Could you check a few things on this model? Use its own coordinates, in mm. Coordinates: 2 decimals unless noted, no trailing zeros. Order: outer loops, then holes, each group sorted by start corner. A loop starts at its lowest first (then second) coordinate and runs counter-clockwise, first axis right, second up. Notation, with made-up numbers: (31.25, 62.25) -> (35.25, 62.25) arc R11 ccw to (35.25, 68.25) -> close; hole circle Ø6 at (-35.75, -1). An arc over 180 degrees is marked (long way). Use a Markdown table: item, result. Add a question column.
1) If we section it at C-C (z = -54.5): Write out the boundary of the cut face in (x, y), plus the area to 3 significant figures.
2) If we section it at B-B (x = 44): Write out the boundary of the cut face in (y, z).
3) If we section it at A-A (y = 0.8): Write out the boundary of the cut face in (x, z).
4) If I drill on L1, parallel to Z at x = 17, y = 1.85; L2, parallel to Z at x = 67.5, y = 2.3; L3, parallel to X at y = 0.5, z = 36.5, over which ranges is the centre line in solid material (lowest first)? Write a range as [from, to].
5) Will these pins go through, and if not, where does the flat tip stop? pin 1 Ø3.5 at (x, z) = (77, 0) entering from +Y; pin 2 Ø2.5 at (x, z) = (-39, 66.39) entering from -Y.
```python
from build123d import *

# Parameters (mm, degrees)
SKETCH1_R           = 75
SKETCH1_R_2         = 73.5
SKETCH1_R_3         = 1.5
BOSS_EXTRUDE1_DEPTH = 2.5


with BuildPart() as part:
    # Sketch1 → Boss-Extrude1 (new body)
    with BuildSketch(Plane(origin=(0, 0, 0), x_dir=(1, 0, 0), z_dir=(0, 1, 0))):
        Circle(SKETCH1_R)
        Circle(SKETCH1_R_2, mode=Mode.SUBTRACT)
        Circle(SKETCH1_R_2)
        with BuildLine():
            ThreePointArc((-65.092339325, -37.255702398), (-75, -1.885e-06), (-65.092341198, 37.255699125))
            ThreePointArc((-65.092341198, 37.255699125), (-73.987141009, 19.120393419), (-80.5, 0))
            ThreePointArc((-80.5, 0), (-73.987140288, -19.120395161), (-65.092339325, -37.255702398))
        make_face()
        with Locations(Location((-77, 0, 0), (0, 0, 270))):
            Circle(SKETCH1_R_3, mode=Mode.SUBTRACT)
        with BuildLine():
            ThreePointArc((-40.772727273, -69.410623904), (-20.577028262, -73.596152049), (5.64e-07, -75))
            ThreePointArc((5.64e-07, -75), (-37.621950265, -64.881344455), (-65.092339325, -37.255702398))
            ThreePointArc((-65.092339325, -37.255702398), (-53.960444579, -54.110599462), (-40.772727273, -69.410623904))
        make_face()
        with Locations(Location((-39, -66.392770691, 0), (0, 0, 270))):
            Circle(SKETCH1_R_3, mode=Mode.SUBTRACT)
        with BuildLine():
            ThreePointArc((40.772727273, -69.410623904), (53.960444658, -54.110599358), (65.092339455, -37.255702172))
            ThreePointArc((65.092339455, -37.255702172), (37.621950865, -64.881344107), (5.64e-07, -75))
            ThreePointArc((5.64e-07, -75), (20.577028821, -73.596151973), (40.772727273, -69.410623904))
        make_face()
        with Locations(Location((39, -66.392770691, 0), (0, 0, 270))):
            Circle(SKETCH1_R_3, mode=Mode.SUBTRACT)
        with BuildLine():
            ThreePointArc((65.092339583, 37.255701948), (72.480774929, 19.27530196), (75, 0))
            ThreePointArc((75, 0), (72.480774896, -19.275302084), (65.092339455, -37.255702172))
            ThreePointArc((65.092339455, -37.255702172), (73.987140338, -19.120395041), (80.5, 0))
            ThreePointArc((80.5, 0), (73.987140387, 19.120394921), (65.092339583, 37.255701948))
        make_face()
        with Locations(Location((77, 0, 0), (0, 0, 270))):
            Circle(SKETCH1_R_3, mode=Mode.SUBTRACT)
        with BuildLine():
            ThreePointArc((-4.58e-07, 75), (37.621950535, 64.881344298), (65.092339583, 37.255701948))
            ThreePointArc((65.092339583, 37.255701948), (53.960444736, 54.110599255), (40.772727273, 69.410623904))
            ThreePointArc((40.772727273, 69.410623904), (20.577028315, 73.596152042), (-4.58e-07, 75))
        make_face()
        with Locations(Location((39, 66.392770691, 0), (0, 0, 270))):
            Circle(SKETCH1_R_3, mode=Mode.SUBTRACT)
        with BuildLine():
            ThreePointArc((-65.092341198, 37.255699125), (-37.621952338, 64.881343253), (-4.58e-07, 75))
            ThreePointArc((-4.58e-07, 75), (-20.577028768, 73.59615198), (-40.772727273, 69.410623904))
            ThreePointArc((-40.772727273, 69.410623904), (-53.960445716, 54.110597958), (-65.092341198, 37.255699125))
        make_face()
        with Locations(Location((-39, 66.392770691, 0), (0, 0, 270))):
            Circle(SKETCH1_R_3, mode=Mode.SUBTRACT)
    extrude(amount=BOSS_EXTRUDE1_DEPTH)


solid = part.part
```
Answer sheet:
| question | item | result |
|---|---|---|
| 1 | outline | (-53.66, 0) -> (53.66, 0) -> (53.66, 2.5) -> (-53.66, 2.5) -> close |
| 1 | area | 268 mm2 |
| 2 | outline | (0, -66.02) -> (2.5, -66.02) -> (2.5, 66.02) -> (0, 66.02) -> close |
| 3 | outline | (-80.5, 0) arc R158.29 ccw to (-40.77, -69.41) arc R151.51 ccw to (40.77, -69.41) arc R158.29 ccw to (80.5, 0) arc R158.29 ccw to (40.77, 69.41) arc R151.51 ccw to (-40.77, 69.41) arc R158.29 ccw to start; hole circle Ø3 at (-77, 0); hole circle Ø3 at (-39, -66.39); hole circle Ø3 at (-39, 66.39); hole circle Ø3 at (39, -66.39); hole circle Ø3 at (39, 66.39); hole circle Ø3 at (77, 0) |
| 4 | L1 | [-74.04, 74.04] |
| 4 | L2 | [-32.89, 32.89] |
| 4 | L3 | [-65.52, 65.52] |
| 5 | pin 1 | y = 2.5 |
| 5 | pin 2 | through |
